Autodesk Inventor part; units mm, degrees
ref_plane "Work Plane1" through (30, 0, 0) normal (1, 0, 0) x (0, 0, -1)
ref_plane "YZ Plane" through (0, 0, 0) normal (1, 0, 0) x (0, 1, 0)
ref_plane "XZ Plane" through (0, 0, 0) normal (0, 1, 0) x (-1, 0, 0)
sketch "Sketch1" plane through (0, 0, 0) normal (0, 1, 0) x (-1, 0, 0)
  line L0 (0, 0) -> (-60, 0)
  line L1 (-60, 0) -> (-60, -70)
  line L2 (-60, -70) -> (0, -70)
  line L3 (0, -70) -> (0, 0)
  dimension "d0" = 60
  dimension "d1" = 70
extrude "Extrusion1" add sketch "Sketch1" along normal blind 12
sketch "Sketch2" plane through (0, 0, 0) normal (0, -1, 0) x (1, 0, 0)
  line L0 (60, -70) -> (0, -70)
  line L1 (60, 0) -> (60, -70)
  line L2 (0, -70) -> (60, -70)
  line L3 (60, -70) -> (60, -65)
  line L4 (60, -65) -> (0, -65)
  line L5 (0, -65) -> (0, -70)
  line L6 (60, 0) -> (57, 0)
  line L7 (57, 0) -> (57, -20)
  line L8 (57, -20) -> (60, -20)
  line L9 (60, -20) -> (60, 0)
  line L10 (0, -70) -> (0, 0)
  line L11 (0, 0) -> (3, 0)
  line L12 (3, 0) -> (3, -20)
  line L13 (3, -20) -> (0, -20)
  line L14 (0, -20) -> (0, 0)
  point P0 (0, -20)
  dimension "d4" = 5
  dimension "d9" = 3
  dimension "d10" = 20
  dimension "d11" = 3
  dimension "d12" = 20
extrude "Extrusion2" add sketch "Sketch2" along normal blind 18
sketch "Sketch3" plane through (60, 0, 0) normal (1, 0, 0) x (0, 0, -1)
  line L0 (65, 0) -> (65, -18)
  line L1 (70, -18) -> (70, 12)
  line L2 (65, -18) -> (70, -18)
  line L3 (70, -18) -> (70, 12)
  line L4 (70, 12) -> (65, 12)
  line L5 (65, 12) -> (65, -18)
  point P0 (0, 0)
extrude "Extrusion3" add sketch "Sketch3" along normal blind 20
ref_plane "Work Plane1" through (30, 0, 0) normal (1, 0, 0) x (0, 0, -1)
mirror "Mirror1" about plane through (30, 0, 0) normal (1, 0, 0) of "Extrusion3"
sketch "Sketch4" plane through (0, 12, 0) normal (0, 1, 0) x (1, 0, 0)
  line L0 (6.5, 38) -> (53.5, 38)
  line L1 (53.5, 38) -> (53.5, 3)
  line L2 (53.5, 3) -> (6.5, 3)
  line L3 (6.5, 3) -> (6.5, 38)
  line L4 (5, 67) -> (26, 67)
  line L5 (26, 67) -> (26, 46)
  line L6 (26, 46) -> (5, 46)
  line L7 (5, 46) -> (5, 67)
  line L8 (31, 63) -> (54, 63)
  line L9 (54, 63) -> (54, 47)
  line L10 (54, 47) -> (31, 47)
  line L11 (31, 47) -> (31, 63)
  line L12 (0, 0) -> (60, 0)
  line L13 (-20, 70) -> (80, 70)
  line L14 (0, 65) -> (0, 0)
  line L15 (60, 0) -> (60, 65)
  point P0 (30, 38)
  point P1 (30, 0)
  dimension "d13" = 47
  dimension "d14" = 35
  dimension "d15" = 21
  dimension "d16" = 21
  dimension "d17" = 23
  dimension "d18" = 16
  dimension "d19" = 3
  dimension "d20" = 7
  dimension "d21" = 3
  dimension "d30" = 5
  dimension "d31" = 6
sketch "Sketch5" plane through (0, 12, 0) normal (0, 1, 0) x (1, 0, 0)
  line L0 (54, 45) -> (6, 45)
  line L1 (5, 44) -> (5, 40)
  line L2 (6, 39) -> (54, 39)
  line L3 (55, 40) -> (55, 44)
  line L4 (26, 46) -> (5, 46)
  line L5 (-20, 70) -> (80, 70)
  line L6 (0, 65) -> (0, 0)
  arc A0 (54, 39) -> (55, 40) centre (54, 40) ccw
  arc A1 (55, 44) -> (54, 45) centre (54, 44) ccw
  arc A2 (6, 45) -> (5, 44) centre (6, 44) ccw
  arc A3 (5, 40) -> (6, 39) centre (6, 40) ccw
  point P0 (55, 45)
  point P1 (5, 39)
  point P2 (55, 39)
  dimension "d22" = 50
  dimension "d23" = 25
  dimension "d24" = 6
  dimension "d25" = 5
  dimension "d26" = 1
  dimension "d27" = 1
extrude "Extrusion4" cut sketch "Sketch5" against normal blind 25
extrude "Extrusion5" cut sketch "Sketch4" against normal blind 10
sketch "Sketch6" plane through (0, 2, 0) normal (0, 1, 0) x (1, 0, 0)
  line L0 (54, 47) -> (31, 47)
  line L1 (54, 63) -> (54, 47)
  line L2 (31, 63) -> (54, 63)
  line L3 (31, 47) -> (31, 63)
  line L4 (33, 61) -> (52, 61)
  line L5 (52, 61) -> (52, 49)
  line L6 (52, 49) -> (33, 49)
  line L7 (33, 49) -> (33, 61)
  point P0 (0, 0)
  dimension "d34" = 2
extrude "Extrusion6" cut sketch "Sketch6" against normal blind 12 contours L4 L5 L6 L7
sketch "Sketch7" plane through (0, 2, 0) normal (0, 1, 0) x (1, 0, 0)
  point P0 (0, 0)
sketch "Sketch8" plane through (0, 2, 0) normal (0, 1, 0) x (1, 0, 0)
  line L0 (26, 46) -> (5, 46)
  line L1 (26, 67) -> (26, 46)
  line L2 (5, 67) -> (26, 67)
  line L3 (5, 46) -> (5, 67)
  point P0 (0, 0)
extrude "Extrusion7" add sketch "Sketch8" along normal blind 4
sketch "Sketch9" plane through (60, 0, -20) normal (1, 0, 0) x (0, 0, -1)
  line L0 (-20, 12) -> (-20, -18)
  line L1 (-20, -18) -> (-12, -18)
  line L2 (-12, -18) -> (-12, 27)
  line L3 (-12, 27) -> (-20, 27)
  line L4 (-20, 27) -> (-20, -18)
  point P0 (-20, 0)
  dimension "d39" = 8
  dimension "d40" = 45
extrude "Extrusion8" add sketch "Sketch9" along normal blind 8
sketch "Sketch10" plane through (3, 0, 0) normal (0, 0, 1) x (1, 0, 0)
  circle A0 centre (61, 23) radius 2.5
  line L0 (57, 27) -> (65, 27)
  point P0 (-3, 0)
  point P1 (61, 27)
  dimension "d43" = 5
  dimension "d44" = 4
extrude "Extrusion9" cut sketch "Sketch10" against normal blind 10
sketch "Sketch12" plane through (68, 0, -20) normal (1, 0, 0) x (0, 0, -1)
  line L0 (-20, 27) -> (-20, -18)
  line L1 (-12, 12) -> (-12, -18)
  line L2 (-20, 17) -> (-12, 17)
  line L3 (-12, 17) -> (-12, 9)
  line L4 (-12, 9) -> (-20, 9)
  line L5 (-20, 9) -> (-20, 17)
  line L6 (-12, 27) -> (-20, 27)
  point P0 (-20, 0)
  dimension "d47" = 10
  dimension "d48" = 8
extrude "Extrusion10" add sketch "Sketch12" along normal blind 8
sketch "Sketch13" plane through (60, 12, -8) normal (0, 0, -1) x (-1, 0, 0)
  circle A0 centre (-12, 1) radius 4
  line L0 (-8, 5) -> (-16, 5)
  line L1 (-16, -3) -> (-16, 5)
  point P0 (60, -12)
  dimension "d51" = 8
extrude "Extrusion11" add sketch "Sketch13" along normal blind 8 contours A0
properties part number "Platform"
Model file for the job. Use its own axes, mm. A direction names the side the tool comes from. Give positions to 0.01 mm unless a question says otherwise; leave off trailing zeros. Write each loop counter-clockwise with the first axis right and the second up, starting at its lowest first coordinate (ties: lowest second). Pieces come first, ordered by that corner, then holes. Notation, with made-up numbers: M 49.5,10.5 L 77.5,10.5 A26 ccw 77.5,31.5 Z; hole C 24,-39 d8. An arc over 180 degrees is marked long. One line per item, written item: value. Start each with the question number.
Q1. Saw through at C-C, the plane y = 23. Write the cut outline in (x, z).
Q2. Saw through at A-A, the plane y = -3.5. Write the cut outline in (x, z), plus the area to 3 significant figures.
Q3. 3-axis set-ups, long thin cutter, end or side, ignore diameter. For faces 4 (the flat face through (3, -9, -10)), 5 (the flat face through (30, 6, -45)), 6 (the flat face through (58, -9, -20)), 7 (the flat face through (31, -7, -65)), 8 (the flat face through (15, 9, -67)): which of +Z, -Z, +X, -X, +Y, -Y reach the whole face in a straight line?
Q4. Saw through at D-D, the plane x = 18. Write the cut outline in (y, z), plus the area to 3 significant figures.
Q5. Saw through at B-B, the plane x = 47. Write the cut outline in (y, z), plus the area to 3 significant figures.
Q6. Two-plate mould, pull along X, no slides. Class faces 1 (the flat face through (52, 1, -55)), 2 (the flat face through (31, -3, -70)), 3 (the flat face through (60, 20, -4)): +X half, -X half, draft (parallel to the pull), parting line (faces both ways), or undercut.
Q7. Drop flat-ended pins along their axis: pin 1 Ø5 at (y, z) = (9.5, -56.5) entering from -X; pin 2 Ø4 at (y, z) = (12.5, -42) entering from +X; pin 3 Ø12 at (x, z) = (10.5, -30.5) entering from -Y. Give the stop position or say it passes through.
Q8. Probe probe 1 along Z at (x, y) = (49, 1.5); probe 2 along Z at (x, y) = (30, 10); probe 3 along Z at (x, y) = (18, 0.5). List the from-to ranges inside material, lowest first. Write a range as [from, to].
Output values:
1. outline: M 60,-8 L 61.5,-8 L 61.5,0 L 60,0 Z; M 66.5,-8 L 68,-8 L 68,0 L 66.5,0 Z
2. outline: M -20,-70 L 80,-70 L 80,-65 L -20,-65 Z; M 0,-20 L 3,-20 L 3,0 L 0,0 Z; M 57,-20 L 60,-20 L 60,-8 L 68,-8 L 68,0 L 57,0 Z
2. area: 684 mm²
3. face 4: +Z, -Y
3. face 5: +Y, -Y
3. face 6: +X, -X, -Y
3. face 7: -Y
3. face 8: +Y
4. outline: M -18,-70 L 12,-70 L 12,-67 L 6,-67 L 6,-46 L 12,-46 L 12,-45 L 0,-45 L 0,-65 L -18,-65 Z; M 0,-39 L 12,-39 L 12,-38 L 2,-38 L 2,-3 L 12,-3 L 12,0 L 0,0 Z
4. area: 382 mm²
5. outline: M -18,-70 L 12,-70 L 12,-63 L 2,-63 L 2,-61 L 0,-61 L 0,-65 L -18,-65 Z; M 0,-49 L 2,-49 L 2,-47 L 12,-47 L 12,-45 L 0,-45 Z; M 0,-39 L 12,-39 L 12,-38 L 2,-38 L 2,-3 L 12,-3 L 12,0 L 0,0 Z
5. area: 324 mm²
6. face 1: undercut
6. face 2: draft
6. face 3: -X half
7. pin 1: stops at x = 0
7. pin 2: stops at x = 60
7. pin 3: stops at y = 0
8. probe 1: z = [-70, -61], [-49, -45], [-39, 0]
8. probe 2: z = [-70, -45], [-39, -38], [-3, 0]
8. probe 3: z = [-70, -45], [-39, 0]
